Could you check a few things on this model? Use its own coordinates, in mm. Face numbers are marked on the shaded views. A direction names the side the tool comes from. Give positions to 0.01 mm unless a question says otherwise; leave off trailing zeros. Loops run counter-clockwise (first coordinate to the right, second up) from the corner with the lowest first, then second, coordinate; pieces in that order, holes last. Notation, with made-up numbers: M 39.5,-24.5 L 49.5,-24.5 A24 ccw 49.5,-4.5 Z; hole C 35,78 d11. An arc over 180 degrees is marked long. Answer in a Markdown table with one row per item. Add a question column.
1. I need wall thicknesses on line 1 along X through (y, z) = (6, 9.75); line 2 along Z through (x, y) = (9, 8). Which ranges of each line are inside material? Lowest first, please. Write a range as from..to.
2. Which directions (+Z, -Z, +X, -X, +Y, -Y) give clear straight access to the entire face, cutting with the end or side of a thin tool? Please do the marked faces 1 and 2.
3. If we section it at C-C on z = 21.5: List the corners of the cut face in (x, y) for me.
4. I'm going to push flat-ended pins straight in: pin 1 Ø3 at (x, y) = (6, 6) entering from +Z; pin 2 Ø2 at (x, y) = (36, 6) entering from -Z; pin 3 Ø10 at (x, z) = (4.5, 15.5) entering from -Y; pin 4 Ø1 at (x, y) = (32.5, 7.5) entering from -Z. Where does each tip first touch, or does it pass through?
5. Thinking about a two-plate mould opening in X: for the marked faces 3, 4 and 5, which applies, released by +X, released by -X, zero draft, split by the parting line, or undercut?
6. If we section it at A-A on y = 21: List the corners of the cut face in (x, z) for me.
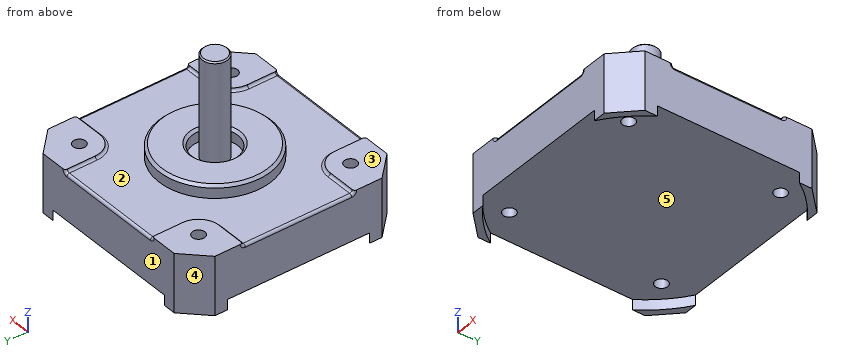
Autodesk Inventor part; units mm, degrees
ref_plane "YZ Plane" through (0, 0, 0) normal (1, 0, 0) x (0, 1, 0)
ref_plane "XZ Plane" through (0, 0, 0) normal (0, 1, 0) x (-1, 0, 0)
ref_plane "XY Plane" through (0, 0, 0) normal (0, 0, 1) x (1, 0, 0)
sketch "Sketch1" plane through (0, 0, 0) normal (0, 0, 1) x (1, 0, 0)
  line L0 (0, 0) -> (42, 0)
  line L1 (42, 0) -> (42, 42)
  line L2 (42, 42) -> (0, 42)
  line L3 (0, 42) -> (0, 0)
  dimension "d0" = 42
  dimension "d1" = 42
extrude "Extrusion1" add sketch "Sketch1" along normal blind 11.5
chamfer "Chamfer1" distance 4.5 angle 45 4 edges at (0, 0, 5.75) (42, 0, 5.75) (42, 42, 5.75) (0, 42, 5.75)
sketch "Sketch2" plane through (0, 0, 11.5) normal (0, 0, 1) x (1, 0, 0)
  line L0 (4.5, 42) -> (37.5, 42)
  line L1 (0, 4.5) -> (0, 37.5)
  line L2 (37.5, 0) -> (4.5, 0)
  line L3 (42, 37.5) -> (42, 4.5)
  line L4 (10, 0) -> (10, 6)
  line L5 (10, 36) -> (10, 42)
  line L6 (0, 32) -> (6, 32)
  line L7 (36, 32) -> (42, 32)
  line L8 (0, 10) -> (6, 10)
  line L9 (36, 10) -> (42, 10)
  line L10 (32, 42) -> (32, 36)
  line L11 (32, 6) -> (32, 0)
  arc A0 (6, 32) -> (10, 36) centre (6, 36) ccw
  arc A1 (32, 36) -> (36, 32) centre (36, 36) ccw
  arc A2 (36, 10) -> (32, 6) centre (36, 6) ccw
  arc A3 (10, 6) -> (6, 10) centre (6, 6) ccw
  dimension "d10" = 4
extrude "Extrusion2" cut sketch "Sketch2" against normal blind 0.5
fillet "Fillet1" radius 0.5 12 edges at (8.8284, 8.8284, 11) (10, 3, 11) (3, 10, 11) (3, 32, 11) (8.8284, 33.1716, 11) (10, 39, 11) (33.1716, 33.1716, 11) (32, 39, 11) (39, 32, 11) (39, 10, 11) (33.1716, 8.8284, 11) (32, 3, 11)
fillet "Fillet2" radius 0.5 12 edges at (0, 21, 11) (0, 10.1463, 11.1463) (0, 31.8537, 11.1463) (21, 42, 11) (10.1463, 42, 11.1463) (31.8537, 42, 11.1463) (42, 21, 11) (42, 31.8537, 11.1463) (42, 10.1463, 11.1463) (21, 0, 11) (31.8537, 0, 11.1463) (10.1463, 0, 11.1463)
sketch "Sketch3" plane through (0, 0, 11) normal (0, 0, 1) x (1, 0, 0)
  circle A0 centre (21, 21) radius 11
  line L0 (10.5, 0) -> (31.5, 0)
  line L1 (0, 31.5) -> (0, 10.5)
  circle A1 centre (21, 21) radius 4.5
  dimension "d15" = 22
  dimension "d16" = 21
  dimension "d17" = 21
  dimension "d18" = 9
extrude "Extrusion3" add sketch "Sketch3" along normal blind 2.5
chamfer "Chamfer2" distance 0.5 angle 45 2 edges at (10, 21, 13.5) (16.5, 21, 13.5)
sketch "Sketch4" plane through (21, 21, 11) normal (0, 0, 1) x (1, 0, 0)
  circle A0 centre (0, 0) radius 4.5
  circle A1 centre (0, 0) radius 2.5
  dimension "d23" = 5
extrude "Extrusion4" add sketch "Sketch4" along normal blind 20 contours A1
sketch "Sketch5" plane through (0, 0, 11.5) normal (0, 0, 1) x (1, 0, 0)
  arc A0 (10, 6) -> (6, 10) centre (6, 6) ccw
  point P0 (36, 6)
  point P1 (6, 36)
  point P2 (36, 36)
  dimension "d28" = 30
  dimension "d29" = 30
hole "Hole1" at (6, 6, 11.5) at (36, 6, 11.5) at (6, 36, 11.5) at (36, 36, 11.5) direction (0, 0, -1) diameter 2.459 end through all
sketch "Sketch6" plane through (0, 0, 0) normal (0, 0, -1) x (-1, 0, 0)
  line L0 (-42, 4.5) -> (-42, 37.5)
  line L1 (-4.5, 0) -> (-37.5, 0)
  circle A0 centre (-21, 21) radius 25.25
  dimension "d37" = 50.5
  dimension "d38" = 21
  dimension "d39" = 21
extrude "Extrusion5" cut sketch "Sketch6" against normal blind 2
chamfer "倒角4" distance 0.25 angle 45 1 edges at (18.5, 21, 31)
properties part number "stepper_front"
Results:
| question | item | result |
|---|---|---|
| 1 | line 1 | 0..4.77, 7.23..34.77, 37.23..42 |
| 1 | line 2 | 2..11.5 |
| 2 | face 1 | +Z, -Z, +X, -X, +Y |
| 2 | face 2 | +Z |
| 3 | outline | C 21,21 d5 |
| 4 | pin 1 | z = 11.5 |
| 4 | pin 2 | through |
| 4 | pin 3 | y = 0 |
| 4 | pin 4 | z = 2 |
| 5 | face 3 | zero draft |
| 5 | face 4 | released by -X |
| 5 | face 5 | undercut |
| 6 | outline | M 0,2 L 42,2 L 42,10.5 A0.5 ccw 41.5,11 L 32,11 L 32,13 L 31.5,13.5 L 26,13.5 L 25.5,13 L 25.5,11 L 23.5,11 L 23.5,30.75 L 23.25,31 L 18.75,31 L 18.5,30.75 L 18.5,11 L 16.5,11 L 16.5,13 L 16,13.5 L 10.5,13.5 L 10,13 L 10,11 L 0.5,11 A0.5 ccw 0,10.5 Z |
